The model under review builds one solid part; all positions refer to its coordinate system, in mm. Face numbers are marked on the shaded views. A direction names the side the tool comes from. Round coordinates to 2 decimals unless told otherwise and drop trailing zeros. Write each loop counter-clockwise with the first axis right and the second up, starting at its lowest first coordinate (ties: lowest second). Pieces come first, ordered by that corner, then holes. Notation, with made-up numbers: (56, 1) -> (79, 1) arc R23 ccw to (79, 33) -> close; hole circle Ø3 at (14.5, 27). An arc over 180 degrees is marked (long way). Answer in a Markdown table with one row per item. Add a question column.
```python
from build123d import *

# Parameters (mm, degrees)
SKETCH1_W                = 42
SKETCH1_H                = 42
BOSS_EXTRUDE1_DEPTH      = 11.6
BOSS_EXTRUDE2_DEPTH      = 5
BOSS_EXTRUDE2_DEPTH_BACK = 18.6
SKETCH2_R                = 2.5


with BuildPart() as part:
    # Sketch1 → Boss-Extrude1 (new body)
    with BuildSketch(Plane.XY):
        Rectangle(SKETCH1_W, SKETCH1_H)
    extrude(amount=BOSS_EXTRUDE1_DEPTH)

    # Sketch2 → Boss-Extrude2 (add, two sides: drawn at the far end of the back side and taken through both)
    with BuildSketch(Plane.XY.offset(11.6).offset(-BOSS_EXTRUDE2_DEPTH_BACK)):
        with Locations(Location((0, 0, 0), (0, 0, 180))):
            Circle(SKETCH2_R)
    extrude(amount=BOSS_EXTRUDE2_DEPTH + BOSS_EXTRUDE2_DEPTH_BACK)


solid = part.part
```
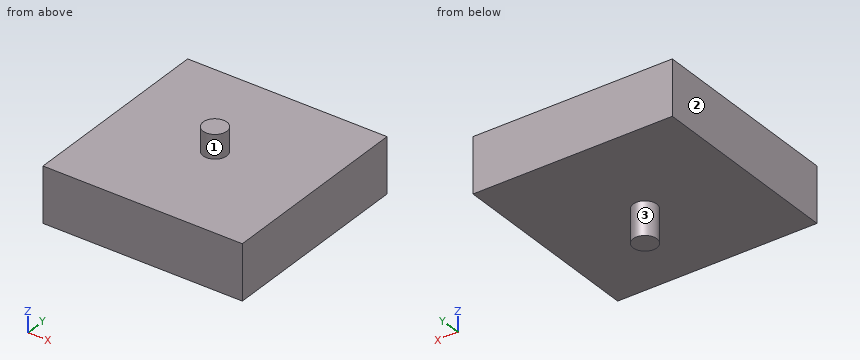
1. Add section A-A on y = -1.5. Write out the cut boundary in (x, z).
2. Add section C-C on z = 12.5. Write out the cut boundary in (x, y).
3. Add section B-B on x = 0. Write out the cut boundary in (y, z), plus the area to 3 significant figures.
4. For L1, parallel to Z at x = -18, y = 13.5; L2, parallel to X at y = -1.5, z = -3, list the stretches that pass through material, from the lowest coordinate up.
5. Insertion check: pin 1 Ø5 at (x, y) = (-2.5, -2.5) entering from -Z; pin 2 Ø3 at (x, y) = (7.5, 8) entering from +Z; pin 3 Ø8 at (x, y) = (-16, 11.5) entering from -Z; pin 4 Ø2 at (x, z) = (8, 14) entering from +Y. Each pin has a flat end and moves straight along its axis. Give the tip position at first contact, or say it passes through.
6. Tool access review of the marked faces 1, 2 and 3: name each direction out of +Z, -Z, +X, -X, +Y, -Y from which nothing blocks a thin tool from reaching the whole face with its end or side.
7. Add section D-D on y = -11. Write out the cut boundary in (x, z).
Filled in:
| question | item | result |
|---|---|---|
| 1 | outline | (-21, 0) -> (-2, 0) -> (-2, -7) -> (2, -7) -> (2, 0) -> (21, 0) -> (21, 11.6) -> (2, 11.6) -> (2, 16.6) -> (-2, 16.6) -> (-2, 11.6) -> (-21, 11.6) -> close |
| 2 | outline | circle Ø5 at (0, 0) |
| 3 | outline | (-21, 0) -> (-2.5, 0) -> (-2.5, -7) -> (2.5, -7) -> (2.5, 0) -> (21, 0) -> (21, 11.6) -> (2.5, 11.6) -> (2.5, 16.6) -> (-2.5, 16.6) -> (-2.5, 11.6) -> (-21, 11.6) -> close |
| 3 | area | 547 mm² |
| 4 | L1 | 0 to 11.6 |
| 4 | L2 | -2 to 2 |
| 5 | pin 1 | z = -7 |
| 5 | pin 2 | z = 11.6 |
| 5 | pin 3 | z = 0 |
| 5 | pin 4 | through |
| 6 | face 1 | +Z |
| 6 | face 2 | +Z, -Z, -X, +Y, -Y |
| 6 | face 3 | -Z |
| 7 | outline | (-21, 0) -> (21, 0) -> (21, 11.6) -> (-21, 11.6) -> close |
